from build123d import *

# Parameters (mm, degrees)
F0_R     = 9.375
F1_DEPTH = 140
F2_DEPTH = 40
F3_COUNT = 3
F0_R_2   = 2.25
F4_DEPTH = 50
F5_START = 62
F0_R_3   = 7.5
F5_DEPTH = 15
F6_R     = 3
F7_DEPTH = 25
F8_R     = 15


with BuildPart() as f1:
    # F0 (on Top) → F1 (new body)
    with BuildSketch(Plane.XY):
        with BuildLine():
            ThreePointArc((3, -9.801147892), (8.2405248619, -6.0955926701), (10.25, 0))
            ThreePointArc((10.25, 0), (7.5083287088, 6.9776428685), (0.75, 10.2225241501))
            ThreePointArc((0.75, 10.2225241501), (0, 10.25), (-0.75, 10.2225241501))
            ThreePointArc((-0.75, 10.2225241501), (-10.185896402, 1.1445586432), (-3, -9.801147892))
            ThreePointArc((-3, -9.801147892), (-1.5166961062, -10.1371659216), (-1.65e-08, -10.25))
            ThreePointArc((-1.65e-08, -10.25), (1.5166960899, -10.137165924), (3, -9.801147892))
        make_face()
        Circle(F0_R, mode=Mode.SUBTRACT)
    extrude(amount=F1_DEPTH)

    # F0 (on Top) → F2 (join)
    with BuildSketch(Plane.XY):
        with BuildLine():
            ThreePointArc((-0.75, 10.2225241501), (0, 10.25), (0.75, 10.2225241501))
            Line((0.75, 10.2225241501), (0.75, 35.2225241501))
            Line((0.75, 35.2225241501), (-0.75, 35.2225241501))
            Line((-0.75, 35.2225241501), (-0.75, 10.2225241501))
        make_face()
    extrude(amount=F2_DEPTH)


with BuildPart() as f3_1:
    # F3: instance of F1
    add(f1.part.rotate(Axis((0, 0, 140), (0, 0, 1)), 1 * 360 / F3_COUNT))


with BuildPart() as f3_2:
    # F3: instance of F1
    add(f1.part.rotate(Axis((0, 0, 140), (0, 0, 1)), 2 * 360 / F3_COUNT))


with BuildPart() as f1_1:
    add(f1.part)

    add(f3_1.part)  # F4 merges F3_1

    add(f3_2.part)  # F4 merges F3_2
    # F0 (on Top) → F4 (join)
    with BuildSketch(Plane.XY):
        with BuildLine():
            ThreePointArc((3, -13.25), (2.1213203377, -11.1286796506), (-1.65e-08, -10.25))
            ThreePointArc((-1.65e-08, -10.25), (-2.1213203494, -11.1286796623), (-3, -13.25))
            ThreePointArc((-3, -13.25), (0, -16.25), (3, -13.25))
        make_face()
        with Locations((0, -13.25)):
            Circle(F0_R_2, mode=Mode.SUBTRACT)
        with BuildLine():
            Line((3, -13.25), (3, -9.801147892))
            ThreePointArc((3, -9.801147892), (1.5166960899, -10.137165924), (-1.65e-08, -10.25))
            ThreePointArc((-1.65e-08, -10.25), (2.1213203377, -11.1286796506), (3, -13.25))
        make_face()
        with BuildLine():
            ThreePointArc((-3, -13.25), (-2.1213203494, -11.1286796623), (-1.65e-08, -10.25))
            ThreePointArc((-1.65e-08, -10.25), (-1.5166961062, -10.1371659216), (-3, -9.801147892))
            Line((-3, -9.801147892), (-3, -13.25))
        make_face()
    extrude(amount=F4_DEPTH)

    # F0 (on Top) → F5 (join)
    with BuildSketch(Plane.XY.offset(F5_START)):
        Circle(F0_R)
        Circle(F0_R_3, mode=Mode.SUBTRACT)
    extrude(amount=F5_DEPTH)

    # F6 (on Front) → F7 (cut)
    with BuildSketch(Plane.XZ):
        with Locations((0, 82.9966113766)):
            Circle(F6_R)
        with Locations((0, 92.9966113766)):
            Circle(F6_R)
    extrude(amount=F7_DEPTH, mode=Mode.SUBTRACT)

    # F8
    f8_edges = [f1_1.edges().sort_by_distance(p)[0] for p in [
        (0, 35.222524, 40),
        (30.503601, -17.611262, 40),
        (-30.503601, -17.611262, 40),
    ]]
    fillet(f8_edges, radius=F8_R)


solid = f1_1.part
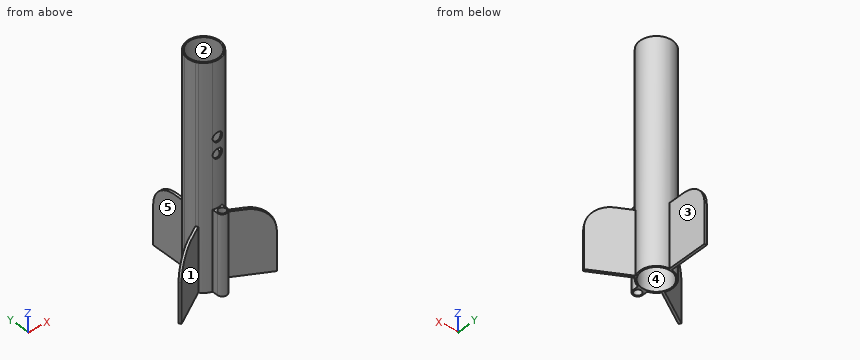
Model file for the job. Use its own axes, mm. Face numbers are marked on the shaded views. A direction names the side the tool comes from. Give positions to 0.01 mm unless a question says otherwise; leave off trailing zeros. Write each loop counter-clockwise with the first axis right and the second up, starting at its lowest first coordinate (ties: lowest second). Pieces come first, ordered by that corner, then holes. Notation, with made-up numbers: M 43,-23 L 92,-23 A18 cw 92,1 Z; hole C -18,89 d2. An arc over 180 degrees is marked long. One line per item, written item: value. Start each with the question number.
Q1. Saw through at B-B, the plane y = 0. Write the cut outline in (x, z) (3 decimals).
Q2. Saw through at A-A, the plane z = 18. State how many separate pieces and enclosed holes the cut face has, plus the area to 3 significant figures.
Q3. Probe probe 1 along Z at (x, y) = (0, -9.5); probe 2 along Y at (x, z) = (0, 16.5) (3 decimals); probe 3 along Y at (x, z) = (0, 117.5) (3 decimals). List the from-to ranges inside material, lowest first. Write a range as [from, to].
Q4. Saw through at D-D, the plane x = -13. Write the cut outline in (y, z), plus the area to 3 significant figures.
Q5. Drop flat-ended pins along their axis: pin 1 Ø12.5 at (y, z) = (28.5, 23.5) entering from +X; pin 2 Ø0.8 at (x, y) = (0.5, 15.5) entering from +Z; pin 3 Ø5 at (x, z) = (0, 83) entering from +Y; pin 4 Ø3.5 at (x, y) = (0, -13.25) entering from -Z. Give the stop position or say it passes through.
Q6. 3-axis set-ups, long thin cutter, end or side, ignore diameter. For the marked faces 1 and 2: which of +Z, -Z, +X, -X, +Y, -Y reach the whole face in a straight line?
Q7. Two-plate mould, pull along X, no slides. Class the marked faces 3, 4 and 5: +X half, -X half, draft (parallel to the pull), parting line (faces both ways), or undercut.
Output values:
1. outline: M -10.25,0 L -9.375,0 L -9.375,62 L -7.5,62 L -7.5,77 L -9.375,77 L -9.375,140 L -10.25,140 Z; M 7.5,62 L 9.375,62 L 9.375,0 L 10.25,0 L 10.25,140 L 9.375,140 L 9.375,77 L 7.5,77 Z
2. separate pieces: 1
2. enclosed holes: 2
2. area: 183 mm²
3. probe 1: z = [0, 80], [86, 90], [96, 140]
3. probe 2: y = [-16.25, -15.5], [-11, -9.375], [9.375, 35.223]
3. probe 3: y = [-10.25, -9.375], [9.375, 10.25]
4. outline: M -8.37,0 L -6.64,0 L -6.64,40 L -8.37,40 Z
4. area: 69.3 mm²
5. pin 1: stops at x = 0.75
5. pin 2: stops at z = 40
5. pin 3: stops at y = 10.25
5. pin 4: passes through
6. face 1: +Z, -Z, -Y
6. face 2: +Z
7. face 3: +X half
7. face 4: undercut
7. face 5: -X half
